Autodesk Inventor part; units mm, degrees
ref_plane "YZ Plane" through (0, 0, 0) normal (1, 0, 0) x (0, 1, 0)
ref_plane "XZ Plane" through (0, 0, 0) normal (0, 1, 0) x (-1, 0, 0)
ref_plane "XY Plane" through (0, 0, 0) normal (0, 0, 1) x (1, 0, 0)
sketch "Sketch2" plane through (0, 0, 0) normal (0, 1, 0) x (-1, 0, 0)
  line L0 (-89, 99) -> (89, 99)
  line L1 (89, 99) -> (89, -99)
  line L2 (89, -99) -> (-89, -99)
  line L3 (-89, -99) -> (-89, 99)
  line L4 (-89, 99) -> (89, -99) construction
  line L5 (89, 99) -> (-89, -99) construction
  line L6 (-89, 99) -> (89, 99)
  line L7 (89, 99) -> (89, -81)
  line L8 (89, -81) -> (-89, -81)
  line L9 (-89, -81) -> (-89, 99)
  line L10 (-4.5, 99) -> (-89, 99)
  line L11 (-89, 99) -> (-89, 43)
  line L12 (-89, 43) -> (-4.5, 43)
  line L13 (-4.5, 43) -> (-4.5, 99)
  line L14 (4.5, 99) -> (89, 99)
  line L15 (89, 99) -> (89, 43)
  line L16 (89, 43) -> (4.5, 43)
  line L17 (4.5, 43) -> (4.5, 99)
  line L18 (22.5, 77.5) -> (22.5, 66.5)
  line L19 (16.5, 66.5) -> (16.5, 77.5)
  line L20 (-22.5, 66.5) -> (-22.5, 77.5)
  line L21 (-16.5, 77.5) -> (-16.5, 66.5)
  line L22 (-23.5, 99) -> (-16.5, 99)
  line L23 (-16.5, 99) -> (-16.5, 43)
  line L24 (-16.5, 43) -> (-23.5, 43)
  line L25 (-23.5, 43) -> (-23.5, 99)
  line L26 (16.5, 99) -> (23.5, 99)
  line L27 (23.5, 99) -> (23.5, 43)
  line L28 (23.5, 43) -> (16.5, 43)
  line L29 (16.5, 43) -> (16.5, 99)
  line L30 (-89, 99) -> (89, 99)
  line L31 (89, 99) -> (89, 98)
  line L32 (89, 98) -> (-89, 98)
  line L33 (-89, 98) -> (-89, 99)
  line L34 (89, -81) -> (74, -81)
  line L35 (74, -81) -> (74, -61)
  line L36 (74, -61) -> (89, -61)
  line L37 (89, -61) -> (89, -81)
  line L38 (-89, -81) -> (-74, -81)
  line L39 (-74, -81) -> (-74, -61)
  line L40 (-74, -61) -> (-89, -61)
  line L41 (-89, -61) -> (-89, -81)
  line L42 (16.5, 98) -> (-16.5, 98)
  line L43 (-16.5, 98) -> (-16.5, 94)
  line L44 (-16.5, 94) -> (16.5, 94)
  line L45 (16.5, 94) -> (16.5, 98)
  line L46 (-84.4, -75) -> (-84.4, -71.5)
  line L47 (-84.4, -71.5) -> (-87, -71.5)
  line L48 (-87, -71.5) -> (-87, -75)
  line L49 (-87, -75) -> (-84.4, -75)
  line L50 (-79.6, -75) -> (-77, -75)
  line L51 (-77, -75) -> (-77, -71.5)
  line L52 (-77, -71.5) -> (-79.6, -71.5)
  line L53 (-79.6, -71.5) -> (-79.6, -75)
  line L54 (-75, -78) -> (-89, -78)
  line L55 (-89, -78) -> (-89, -63)
  line L56 (-89, -63) -> (-75, -63)
  line L57 (-75, -63) -> (-75, -78)
  circle A0 centre (-80.45, -67.25) radius 1.25
  point P0 (0, 0)
  point P1 (4.5, 99)
  point P2 (-4.5, 99)
  point P3 (-89, 43)
  point P4 (89, 43)
  point P5 (4.5, 98)
  point P6 (-4.5, 98)
  point P7 (-16.5, 98)
  point P8 (-23.5, 98)
  point P9 (23.5, 98)
  point P10 (16.5, 98)
  point P11 (-4.5, 94)
  point P12 (4.5, 94)
  point P13 (16.5, 94)
  dimension "d8" = 178
  dimension "d9" = 198
  dimension "d10" = 18
  dimension "d11" = 84.5
  dimension "d13" = 84.5
  dimension "d17" = 9
  dimension "d18" = 1
  dimension "d19" = 15
  dimension "d20" = 20
  dimension "d21" = 15
  dimension "d22" = 20
  dimension "d75" = 55
  dimension "d76" = 55
  dimension "d77" = 7
  dimension "d78" = 7
  dimension "d79" = 4
extrude "Extrusion2" add sketch "Sketch2" along normal blind 3 contours L32 L23 L21 L12 L25 | L12 L13 L44 L17 L16 L1 L36 L35 L8 L39 L40 L3 | L32 L13 L44 L23 | L32 L17 L44 L13 | L32 L29 L44 L17 | L32 L27 L16 L29 L19
equation "\"d11\" = d13"
properties part number "base" material "Aluminum 6061"
Input: part model. Units: mm. Frame: model coordinates. Coordinates: 2 decimals unless noted, no trailing zeros. Loops run counter-clockwise (first coordinate to the right, second up) from the corner with the lowest first, then second, coordinate; pieces in that order, holes last. Notation, with made-up numbers: (52.5, 69) - (59.5, 69) arc R24 ccw to (59.5, 86) - close; hole circle Ø9 at (1, 89). An arc over 180 degrees is marked (long way). Answer in a Markdown table with one row per item.
(1) Cut plane B-B on z = 73. Output: boundary loops of the cut face in (x, y).
Model answer:
| item | result |
|---|---|
| outline | (-23.5, 0) - (-16.5, 0) - (-16.5, 3) - (-23.5, 3) - close; (-4.5, 0) - (4.5, 0) - (4.5, 3) - (-4.5, 3) - close; (16.5, 0) - (23.5, 0) - (23.5, 3) - (16.5, 3) - close |
(2) Pin query (flat end, axial travel): P1, Ø0.9, axis at x = 56, y = 2, coming from the +Z side; P2, Ø0.9, axis at y = 1, z = -68.5, coming from the -X side; P3, Ø1.5, axis at x = 81, y = 1, coming from the -Z side. Return the tip coordinate at first contact, or that it passes through.
Model answer:
| item | result |
|---|---|
| P1 | stops at z = 43 |
| P2 | stops at x = -74 |
| P3 | stops at z = -61 |
(3) Material intervals for L1, parallel to X at y = 0.5, z = 77; L2, parallel to Z at x = 14, y = 2.15; L3, parallel to Z at x = 31.5, y = 0.45, sorted ascending. Write a range as from..to.
Model answer:
| item | result |
|---|---|
| L1 | x = -23.5..-16.5, -4.5..4.5, 16.5..23.5 |
| L2 | z = -81..43, 94..98 |
| L3 | z = -81..43 |
(4) Cut plane A-A on y = 2.3. Output: boundary loops of the cut face in (x, z).
Model answer:
| item | result |
|---|---|
| outline | (-89, -61) - (-74, -61) - (-74, -81) - (74, -81) - (74, -61) - (89, -61) - (89, 43) - (23.5, 43) - (23.5, 98) - (-23.5, 98) - (-23.5, 43) - (-89, 43) - close; hole (-16.5, 43) - (-4.5, 43) - (-4.5, 94) - (-16.5, 94) - close; hole (4.5, 43) - (16.5, 43) - (16.5, 94) - (4.5, 94) - close |
(5) Cut plane C-C on x = -71. Output: boundary loops of the cut face in (y, z).
Model answer:
| item | result |
|---|---|
| outline | (0, -81) - (3, -81) - (3, 43) - (0, 43) - close |
